Source: CAD feature listing. Evaluate the final solid. Frame: model axes, mm. Face numbers are marked on the shaded views. Coordinates: 2 decimals unless noted, no trailing zeros. Loops run counter-clockwise (first coordinate to the right, second up) from the corner with the lowest first, then second, coordinate; pieces in that order, holes last. Notation, with made-up numbers: (-23, 23) -> (25, 23) arc R33 ccw to (25, 62) -> close; hole circle Ø6 at (24, 4.25). An arc over 180 degrees is marked (long way). Answer as CSV lines item,"result".
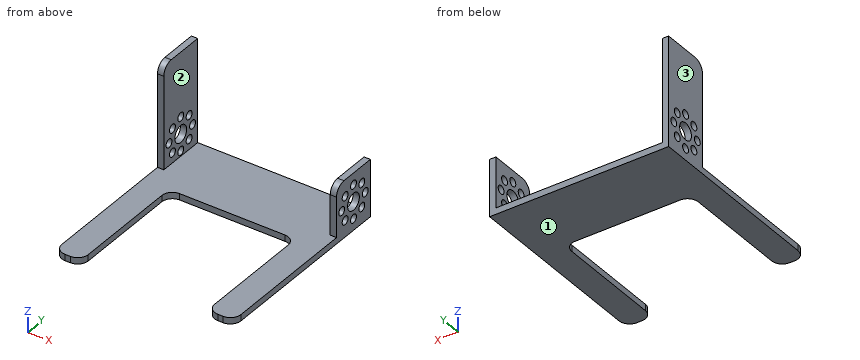
from build123d import *

# Parameters (mm, degrees)
F0_W     = 85
F0_H     = 23
F1_DEPTH = 3
F2_W     = 3
F2_H     = 23
F3_DEPTH = 24
F4_W     = 3
F4_H     = 23
F5_DEPTH = 25
F6_R     = 4
F6_R_2   = 2
F7_DEPTH = 100
F8_R     = 5


with BuildPart() as f1:
    # F0 (on Top) → F1 (new body)
    with BuildSketch(Plane.XY):
        with Locations((42.5, 11.5)):
            Rectangle(F0_W, F0_H)
        with BuildLine():
            Line((85, 0), (0, 0))
            Line((0, 0), (0, -10))
            Line((0, -10), (0, -65))
            ThreePointArc((0, -65), (1.464466, -68.535534), (5, -70))
            Line((5, -70), (7.5, -70))
            ThreePointArc((7.5, -70), (11.035534, -68.535534), (12.5, -65))
            Line((12.5, -65), (12.5, -15))
            ThreePointArc((12.5, -15), (13.964466, -11.464466), (17.5, -10))
            Line((17.5, -10), (67.5, -10))
            ThreePointArc((67.5, -10), (71.035534, -11.464466), (72.5, -15))
            Line((72.5, -15), (72.5, -65))
            ThreePointArc((72.5, -65), (73.964466, -68.535534), (77.5, -70))
            Line((77.5, -70), (80, -70))
            ThreePointArc((80, -70), (83.535534, -68.535534), (85, -65))
            Line((85, -65), (85, -10))
            Line((85, -10), (85, 0))
        make_face()
    extrude(amount=F1_DEPTH)

    # F2 (on face) → F3 (join)
    with BuildSketch(Plane.XY.offset(3)):
        with Locations((1.5, 11.5)):
            Rectangle(F2_W, F2_H)
        with Locations((83.5, 11.5)):
            Rectangle(F2_W, F2_H)
    extrude(amount=F3_DEPTH)

    # F4 (on face) → F5 (join)
    with BuildSketch(Plane.XY.offset(27)):
        with Locations((1.5, 11.5)):
            Rectangle(F4_W, F4_H)
    extrude(amount=F5_DEPTH)

    # F6 (on face) → F7 (cut)
    with BuildSketch(Plane.YZ.offset(85)):
        with Locations((11.5, 13.5)):
            Circle(F6_R)
        with Locations((19.5, 13.5)):
            Circle(F6_R_2)
        with Locations((17.156854, 19.156854)):
            Circle(F6_R_2)
        with Locations((11.5, 21.5)):
            Circle(F6_R_2)
        with Locations((5.843146, 19.156854)):
            Circle(F6_R_2)
        with Locations((3.5, 13.5)):
            Circle(F6_R_2)
        with Locations((5.843146, 7.843146)):
            Circle(F6_R_2)
        with Locations((11.5, 5.5)):
            Circle(F6_R_2)
        with Locations((17.156854, 7.843146)):
            Circle(F6_R_2)
    extrude(amount=-F7_DEPTH, mode=Mode.SUBTRACT)

    # F8
    f8_edges = [f1.edges().sort_by_distance(p)[0] for p in [
        (1.5, 0, 52),
        (83.5, 0, 27),
    ]]
    fillet(f8_edges, radius=F8_R)


solid = f1.part
(1) Cut plane C-C (y = -22.5). Return the cut outline in (x, z).
Computed values:
outline,"(0, 0) -> (12.5, 0) -> (12.5, 3) -> (0, 3) -> close; (72.5, 0) -> (85, 0) -> (85, 3) -> (72.5, 3) -> close"
(2) Pin query (flat end, axial travel): pin 1 Ø1.5 at (y, z) = (10.5, 22) entering from -X; pin 2 Ø2.5 at (x, z) = (50.5, 1.5) entering from -Y. Return the tip coordinate at first contact, or that it passes through.
Computed values:
pin 1,"through"
pin 2,"y = -10"
(3) Cut plane D-D (x = 31). Return the cut outline in (y, z), then the cut area to 3 significant figures.
Computed values:
outline,"(-10, 0) -> (23, 0) -> (23, 3) -> (-10, 3) -> close"
area,"99.0 mm^2"
(4) Draft query along X for the marked faces 1, 2 and 3. Return one class per face: released by +X, released by -X, zero draft, split by the parting line, or undercut.
Computed values:
face 1,"zero draft"
face 2,"undercut"
face 3,"released by -X"
(5) Material intervals for L1, parallel to Z at x = 84, y = 11.5; L2, parallel to Z at x = 2, y = 11.5; L3, parallel to Z at x = 4, y = -26, sorted ascending. Write a range as [from, to].
Computed values:
L1,"[0, 3.5], [7.5, 9.5], [17.5, 19.5], [23.5, 27]"
L2,"[0, 3.5], [7.5, 9.5], [17.5, 19.5], [23.5, 52]"
L3,"[0, 3]"
(6) Cut plane A-A (y = 11.5). State how many separate pieces and enclosed holes the cut face has, then the cut area to 3 significant figures.
Computed values:
separate pieces,"7"
enclosed holes,"0"
area,"378 mm^2"
